Can you work these out from the drawing? Everything is in mm from the part's minimum corner. A direction names the side the tool comes from. Coordinates: 2 decimals unless noted, no trailing zeros. Write each loop counter-clockwise with the first axis right and the second up, starting at its lowest first coordinate (ties: lowest second). Pieces come first, ordered by that corner, then holes. Notation, with made-up numbers: (24.5, 36.25) -> (43.5, 36.25) arc R26 ccw to (43.5, 68.25) -> close; hole circle Ø1 at (78.25, 81). An arc over 180 degrees is marked (long way). Answer as CSV lines item,"result". Start each with the question number.
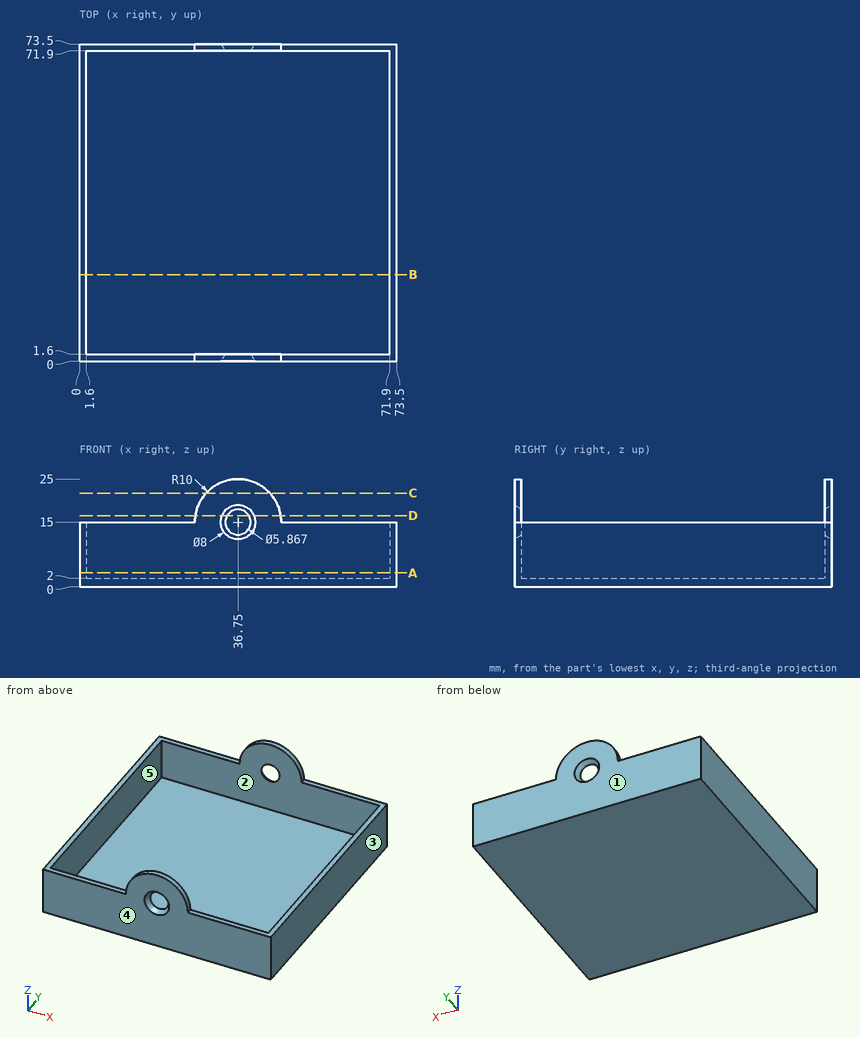
Q1. Imagine slicing it at B-B (y = 20). Write out the boundary of the cut face in (x, z).
Q2. For pin 1 (1.5 mm diameter, centred on x = 9.5, y = 66, fed in from +Z); pin 2 (21.5 mm diameter, centred on x = 66, y = 52, fed in from +Z), each with a flat end and sliding along its axis, tell me the tip position at first contact or that it passes through.
Q3. Which directions (+Z, -Z, +X, -X, +Y, -Y) give clear straight access to the entire face, cutting with the end or side of a thin tool? Please do the marked faces 1 and 2.
Q4. Imagine slicing it at C-C (z = 21.75). Write out the boundary of the cut face in (x, y).
Q5. Imagine slicing it at D-D (z = 16.5). State how many separate pieces and enclosed holes the cut face has, then the cut area to 3 significant figures.
Q6. I need wall thicknesses on L1, parallel to Y at x = 70, z = 2.5; L2, parallel to Z at x = 41, y = 41.5. Which ranges of each line are inside material? Lowest first, please.
Q7. Imagine slicing it at A-A (z = 3.25). Write out the boundary of the cut face in (x, y).
Q8. If we mould it in two halves opening along Y, with no side actions, what happens to the marked faces 3, 4 and 5? For each: released by +Y, released by -Y, zero draft, split by the parting line, or undercut.
Entries:
1,outline,"(0, 0) -> (73.5, 0) -> (73.5, 15) -> (71.9, 15) -> (71.9, 2) -> (1.6, 2) -> (1.6, 15) -> (0, 15) -> close"
2,pin 1,"z = 2"
2,pin 2,"z = 15"
3,face 1,"+Z, -Z, +X, -X, +Y"
3,face 2,"+Z"
4,outline,"(29.37, 0) -> (44.13, 0) -> (44.13, 1.6) -> (29.37, 1.6) -> close; (29.37, 71.9) -> (44.13, 71.9) -> (44.13, 73.5) -> (29.37, 73.5) -> close"
5,separate pieces,"4"
5,enclosed holes,"0"
5,area,"43.3 mm2"
6,L1,"0 to 1.6, 71.9 to 73.5"
6,L2,"0 to 2"
7,outline,"(0, 0) -> (73.5, 0) -> (73.5, 73.5) -> (0, 73.5) -> close; hole (1.6, 1.6) -> (71.9, 1.6) -> (71.9, 71.9) -> (1.6, 71.9) -> close"
8,face 3,"zero draft"
8,face 4,"released by -Y"
8,face 5,"undercut"
